```python
from build123d import *

# Parameters (mm, degrees)
BOSS_EXTRUDE1_DEPTH = 127
CUT_EXTRUDE1_DEPTH  = 127
CUT_EXTRUDE2_DEPTH  = 127
CUT_EXTRUDE3_DEPTH  = 127
CUT_EXTRUDE4_DEPTH  = 127
CUT_EXTRUDE5_DEPTH  = 35.56
CUT_EXTRUDE6_DEPTH  = 45.72
CUT_EXTRUDE7_DEPTH  = 25.4
CUT_EXTRUDE8_DEPTH  = 25.4
CUT_EXTRUDE9_DEPTH  = 48.26
FILLET2_R           = 12.7
CUT_EXTRUDE10_DEPTH = 48.26
CUT_EXTRUDE11_DEPTH = 48.26
SKETCH13_W          = 3.352326168
SKETCH13_H          = 6.321243204
SKETCH13_W_2        = 2.726283313
SKETCH13_W_3        = 3.104310258
CUT_EXTRUDE12_DEPTH = 48.26


with BuildPart() as part:
    # Sketch1 → Boss-Extrude1 (new body)
    with BuildSketch(Plane(origin=(0, 0, 0), x_dir=(1, 0, 0), z_dir=(0, 1, 0))):
        with BuildLine():
            Line((-46.648149315, -23.52267691), (-46.648149315, -48.412154961))
            Line((-46.648149315, -48.412154961), (-40.062268629, -48.412154961))
            ThreePointArc((-40.062268629, -48.412154961), (-28.224090342, -53.116170018), (-16.385912055, -48.412154961))
            Line((-16.385912055, -48.412154961), (82.712264752, -48.412154961))
            Line((82.712264752, -48.412154961), (82.712264752, 45.668146178))
            Line((82.712264752, 45.668146178), (82.57362293, 45.668146178))
            ThreePointArc((82.57362293, 45.668146178), (49.392158098, 86.647568698), (16.210693266, 45.668146178))
            Line((16.210693266, 45.668146178), (-46.648149315, 45.668146178))
            Line((-46.648149315, 45.668146178), (-46.648149315, 20.778668127))
            ThreePointArc((-46.648149315, 20.778668127), (-57.035515889, -1.372004392), (-46.648149315, -23.52267691))
        make_face()
    extrude(amount=BOSS_EXTRUDE1_DEPTH)

    # Sketch2 → Cut-Extrude1 (cut)
    with BuildSketch(Plane(origin=(0, 127, 0), x_dir=(1, 0, 0), z_dir=(0, 1, 0))):
        Polygon((53.771255125, -48.412154961), (53.771255125, -33.133056701), (59.245344615, -38.607146191), (64.805708774, -15.565956225), (67.56040543, -24.817995886), (71.210896888, -21.167504428), (74.240128171, -27.086551208), (78.610346891, -31.456769928), (82.712264752, -27.354852067), (82.712264752, -48.412154961), align=None)
    extrude(amount=-CUT_EXTRUDE1_DEPTH, mode=Mode.SUBTRACT)

    # Sketch3 → Cut-Extrude2 (cut)
    with BuildSketch(Plane(origin=(0, 127, 0), x_dir=(1, 0, 0), z_dir=(0, 1, 0))):
        Polygon((-54.021260569, 11.457814404), (-48.290157028, 8.607539769), (-56.529413656, 4.004510667), (-59.573272313, 8.607539769), align=None)
    extrude(amount=-CUT_EXTRUDE2_DEPTH, mode=Mode.SUBTRACT)

    # Sketch4 → Cut-Extrude3 (cut)
    with BuildSketch(Plane(origin=(0, 127, 0), x_dir=(1, 0, 0), z_dir=(0, 1, 0))):
        Polygon((68.711913571, 80.608646732), (61.499352783, 77.062236982), (61.499352783, 84.413487152), (43.506651189, 77.062236982), (37.732058212, 79.486880591), (37.732058212, 73.421951288), (29.019187448, 73.421951288), (32.795774648, 59.641721258), (25.052672929, 57.519659523), (23.039136033, 52.724168763), (15.468758164, 52.724168763), (7.703729169, 71.729623121), (36.607461416, 93.948488974), (52.503001986, 98.304794706), (65.105633177, 93.013185532), (69.999007684, 86.647568698), align=None)
    extrude(amount=-CUT_EXTRUDE3_DEPTH, mode=Mode.SUBTRACT)

    # Sketch5 → Cut-Extrude4 (cut)
    with BuildSketch(Plane.XY.offset(48.412154961)):
        Polygon((23.551684909, 96.675783769), (33.794948234, 86.432520444), (19.119619253, 71.757191462), (0, 79.094855953), (0, 101.828672261), (14.231003477, 87.597668784), align=None)
    extrude(amount=-CUT_EXTRUDE4_DEPTH, mode=Mode.SUBTRACT)

    # Sketch6 → Cut-Extrude5 (cut)
    with BuildSketch(Plane.ZY.offset(46.648149315)):
        Polygon((38.182028022, 0), (33.400703039, 7.024347662), (37.217405556, 9.622296393), (35.309054298, 16.783843232), (38.182028022, 16.783843232), (40.605664491, 14.360206762), (44.842860178, 18.597402448), (44.842860178, 22.591859045), (48.412154961, 19.022564262), (59.012556324, 19.022564262), (59.012556324, 0), (48.412154961, 0), align=None)
    extrude(amount=-CUT_EXTRUDE5_DEPTH, mode=Mode.SUBTRACT)

    # Sketch7 → Cut-Extrude6 (cut)
    with BuildSketch(Plane.XY.offset(48.412154961)):
        Polygon((39.132383475, 25.016517963), (28.526826147, 14.410960635), (36.827561927, 6.110224855), (40.977929817, 10.260592745), (36.827561927, 14.410960635), align=None)
    extrude(amount=-CUT_EXTRUDE6_DEPTH, mode=Mode.SUBTRACT)

    # Sketch8 → Cut-Extrude7 (cut)
    with BuildSketch(Plane(origin=(0, 127, 0), x_dir=(1, 0, 0), z_dir=(0, 1, 0))):
        with BuildLine():
            Line((-57.002829821, 0), (-49.785263054, 0))
            Line((-49.785263054, 0), (-52.666628039, -16.625220216))
            ThreePointArc((-52.666628039, -16.625220216), (-57.55914693, -15.494773831), (-62.296457645, -13.829680042))
            Line((-62.296457645, -13.829680042), (-57.002829821, 0))
        make_face()
    extrude(amount=-CUT_EXTRUDE7_DEPTH, mode=Mode.SUBTRACT)

    # Sketch9 → Cut-Extrude8 (cut)
    with BuildSketch(Plane.XZ):
        Polygon((82.712264752, 0), (39.607419236, -9.156647056), (54.793750982, -19.021436188), (48.928269368, -28.051041225), (61.159841994, -35.996467858), (82.712264752, -19.021436188), align=None)
    extrude(amount=-CUT_EXTRUDE8_DEPTH, mode=Mode.SUBTRACT)

    # Sketch10 → Cut-Extrude9 (cut)
    with BuildSketch(Plane.XY.offset(48.412154961)):
        Polygon((53.771255125, 107.29121559), (42.256216165, 102.017164953), (46.287188011, 98.336825396), (46.287188011, 93.216188047), (49.045405549, 90.697892831), (50.235317507, 84.59608405), (48.703232752, 82.918034942), (53.771255125, 78.290852235), (61.466936814, 80.968679424), (67.014073164, 73.774503757), (72.871402474, 78.290852235), (77.043238703, 83.646506612), (69.697413806, 84.59608405), (76.045391143, 89.490751273), (72.68469634, 93.849293635), (77.043238703, 97.209988438), (68.326153978, 98.336825396), (66.050570011, 103.030602234), align=None)
    extrude(amount=-CUT_EXTRUDE9_DEPTH, mode=Mode.SUBTRACT)

    # Fillet2
    fillet2_edges = [part.edges().sort_by_distance(p)[0] for p in [
        (-15.218728024, 0, -45.668146178),
    ]]
    fillet(fillet2_edges, radius=FILLET2_R)

    # Sketch11 → Cut-Extrude10 (cut)
    with BuildSketch(Plane(origin=(0, 127, 0), x_dir=(1, 0, 0), z_dir=(0, 1, 0))):
        Polygon((-33.561061306, 45.668146178), (-37.667043384, 39.545827315), (-38.873955148, 45.668146178), align=None)
    extrude(amount=-CUT_EXTRUDE10_DEPTH, mode=Mode.SUBTRACT)

    # Sketch12 → Cut-Extrude11 (cut)
    with BuildSketch(Plane(origin=(0, 127, 0), x_dir=(1, 0, 0), z_dir=(0, 1, 0))):
        with BuildLine():
            Line((32.62261169, 23.954039897), (0, 11.47123499))
            Line((0, 11.47123499), (11.785114171, 6.209119257))
            ThreePointArc((11.785114171, 6.209119257), (14.943546446, 1.324840992), (19.768883298, -1.922926376))
            Line((19.768883298, -1.922926376), (19.768883298, -9.559025438))
            Line((19.768883298, -9.559025438), (32.25248958, 2.120086108))
            ThreePointArc((32.25248958, 2.120086108), (25.311240294, 13.407729102), (36.117063667, 21.077540525))
            ThreePointArc((36.117063667, 21.077540525), (34.482898742, 22.653139956), (32.62261169, 23.954039897))
        make_face()
        with BuildLine():
            Line((44.311200133, 13.401683946), (44.859521729, 13.914669452))
            ThreePointArc((44.859521729, 13.914669452), (44.41506933, 14.350797491), (43.935008387, 14.747391861))
            ThreePointArc((43.935008387, 14.747391861), (44.147380403, 14.081324283), (44.311200133, 13.401683946))
        make_face()
        with BuildLine():
            ThreePointArc((36.497852258, 2.312544405), (39.537766596, 8.935870024), (38.967288817, 16.201135094))
            ThreePointArc((38.967288817, 16.201135094), (32.362672824, 10.211625014), (36.497852258, 2.312544405))
        make_face()
    extrude(amount=-CUT_EXTRUDE11_DEPTH, mode=Mode.SUBTRACT)

    # Sketch13 → Cut-Extrude12 (cut)
    with BuildSketch(Plane.XY.offset(48.412154961)):
        with Locations((-13.231710861, 123.839378398)):
            Rectangle(SKETCH13_W, SKETCH13_H)
        with Locations((-7.25167366, 123.839378398)):
            Rectangle(SKETCH13_W_2, SKETCH13_H)
        with Locations((-1.552155129, 123.839378398)):
            Rectangle(SKETCH13_W_3, SKETCH13_H)
        Polygon((2.732268262, 127), (4.714756247, 127), (4.714756247, 118.574601007), align=None)
    extrude(amount=-CUT_EXTRUDE12_DEPTH, mode=Mode.SUBTRACT)


solid = part.part
```
Can you work these out from the model? Positions are in its coordinate system, mm. A direction names the side the tool comes from. Give positions to 0.01 mm unless a question says otherwise; leave off trailing zeros. Order: outer loops, then holes, each group sorted by start corner. A loop starts at its lowest first (then second) coordinate and runs counter-clockwise, first axis right, second up. Notation, with made-up numbers: M -29.75,77 L -4.75,77 A4 ccw -4.75,83 Z; hole C 44.5,48.5 d4. An arc over 180 degrees is marked long. Write item = value, one per line. Start each with the question number.
Q1. For faces 3 (the flat face through (40.66, 64.389, -78.258)), 4 (the flat face through (30.86, 80.6, -23.28)), 5 (the flat face through (-3.104, 124, 25)), 6 (the flat face through (18.826, 92.073, -35.172)), 7 (the flat face through (-29.117, 8.305, 35.282)), which set-ups out of +Z, -Z, +X, -X, +Y, -Y let a thin tool reach every point of the face, with its end or its side?
Q2. We'd pull the mould along Y, two halves only. Please class faces 1 (the flat face through (74.928, 80.931, 15.229)), 2 (the flat face through (61.462, 12.522, -4.514)): pulls with the +Y half, pulls with the -Y half, needs draft (parallel to the pull), parting line crosses it, or undercut.
Q3. Suppose I cut it at C-C (y = 109.5). Count the separate pieces of the cut face and the enclosed holes in it, plus the area to 3 significant figures.
Q4. I need wall thicknesses on probe 1 along Z at (x, y) = (-41.5, 61); probe 2 along Y at (x, z) = (24.5, 11.5); probe 3 along Y at (x, z) = (56, 20.5). Which ranges of each line are inside material? Lowest first, please. Write a range as [from, to].
Q5. Suppose I cut it at B-B (z = -62.5). Write out the boundary of the cut face in (x, y), plus the area to 3 significant figures.
Q6. Will these pins go through, and if not, where does the flat tip stop? pin 1 Ø7.5 at (y, z) = (24, 42.5) entering from +X; pin 2 Ø12.5 at (y, z) = (92, 37) entering from -X; pin 3 Ø8 at (y, z) = (90.5, 15.5) entering from +X.
Check result:
q1.face_3 = -Z, +Y, -Y
q1.face_4 = +Y
q1.face_5 = +Z, +Y
q1.face_6 = +Z, -Z
q1.face_7 = +Z, -X
q2.face_1 = undercut
q2.face_2 = needs draft
q3.separate_pieces = 1
q3.enclosed_holes = 3
q3.area = 13,100 mm2
q4.probe_1 = [-45.67, 48.41]
q4.probe_2 = [0, 77.14], [95.73, 127]
q4.probe_3 = [0, 79.07], [106.52, 127]
q5.outline = M 32.01,0 L 81.88,0 L 81.88,127 L 32.01,127 L 32.01,88.22 L 33.79,86.43 L 32.01,84.65 Z
q5.area = 6,330 mm2
q6.pin_1 = 53.77
q6.pin_2 = -46.65
q6.pin_3 = 82.71
